The model under review builds one solid part; all positions refer to its coordinate system, in mm. Round coordinates to 2 decimals unless told otherwise and drop trailing zeros. Write each loop counter-clockwise with the first axis right and the second up, starting at its lowest first coordinate (ties: lowest second). Pieces come first, ordered by that corner, then holes. Notation, with made-up numbers: (48.5, -28) - (89.5, -28) arc R34 cw to (89.5, 4) - close; hole circle Ø2 at (19, 31.5). An arc over 180 degrees is marked (long way). Return JSON: item names as keys, results as strings.
from build123d import *

# Parameters (mm, degrees)
F0_R     = 17.5
F0_R_2   = 4.1
F0_R_3   = 3.375
F1_DEPTH = 10.75
F2_SIZE  = 3


with BuildPart() as f1:
    # F0 (on Top) → F1 (new body)
    with BuildSketch(Plane.XY):
        Circle(F0_R)
        with Locations((0, -8.725)):
            Circle(F0_R_2, mode=Mode.SUBTRACT)
        with Locations((-8.725, 0)):
            Circle(F0_R_3, mode=Mode.SUBTRACT)
        with Locations((8.725, 0)):
            Circle(F0_R_3, mode=Mode.SUBTRACT)
        with Locations((0, 8.725)):
            Circle(F0_R_2, mode=Mode.SUBTRACT)
    extrude(amount=F1_DEPTH)

    # F2
    f2_edges = [f1.edges().sort_by_distance(p)[0] for p in [
        (-4.1, 8.725, 10.75),
        (-4.1, -8.725, 10.75),
    ]]
    chamfer(f2_edges, length=F2_SIZE)


solid = f1.part
(1) Mouldability with a two-part tool opening along Y and no side actions: class faces 1 (the cylindrical face through (-0.889, 4.722, 3.821)), 2 (the flat face through (0, 0, 0)), 3 (the cylindrical face through (-5.5, 1, 5.3)), 4 (the cylindrical face through (-13.887, -10.648, 5.3)) as released by +Y, released by -Y, zero draft, split by the parting line, or undercut.
Filled in:
{"face 1": "undercut", "face 2": "zero draft", "face 3": "undercut", "face 4": "split by the parting line"}
(2) Add section C-C (x = 11). Write out the cut boundary in (y, z).
Filled in:
{"outline": "(-13.61, 0) - (-2.49, 0) - (-2.49, 10.75) - (-13.61, 10.75) - close; (2.49, 0) - (13.61, 0) - (13.61, 10.75) - (2.49, 10.75) - close"}
(3) Wall thickness on line 1 (Y direction, x = 0, z = 2.25) (3 decimals); line 2 (X direction, y = -0.5, z = 7.5); line 3 (X direction, y = -1.5, z = 3.25): over which ranges is each line inside the solid? List them lowest first.
Filled in:
{"line 1": "y = -17.5 to -12.825, -4.625 to 4.625, 12.825 to 17.5", "line 2": "x = -17.49 to -12.06, -5.39 to 5.39, 12.06 to 17.49", "line 3": "x = -17.44 to -11.75, -5.7 to 5.7, 11.75 to 17.44"}
(4) Add section D-D (z = 3.5). Write out the cut boundary in (x, y) (3 decimals), plus the area to 3 significant figures.
Filled in:
{"outline": "circle Ø35 at (0, 0); hole circle Ø6.75 at (-8.725, 0); hole circle Ø8.2 at (0, -8.725); hole circle Ø8.2 at (0, 8.725); hole circle Ø6.75 at (8.725, 0)", "area": "785 mm2"}
(5) Add section A-A (x = 0). Write out the cut boundary in (y, z) (3 decimals), plus the area to 3 significant figures.
Filled in:
{"outline": "(-17.5, 0) - (-12.825, 0) - (-12.825, 7.75) - (-15.825, 10.75) - (-17.5, 10.75) - close; (-4.625, 0) - (4.625, 0) - (4.625, 7.75) - (1.625, 10.75) - (-1.625, 10.75) - (-4.625, 7.75) - close; (12.825, 0) - (17.5, 0) - (17.5, 10.75) - (15.825, 10.75) - (12.825, 7.75) - close", "area": "182 mm2"}
(6) Add section B-B (y = 0). Write out the cut boundary in (x, z), plus the area to 3 significant figures.
Filled in:
{"outline": "(-17.5, 0) - (-12.1, 0) - (-12.1, 10.75) - (-17.5, 10.75) - close; (-5.35, 0) - (5.35, 0) - (5.35, 10.75) - (-5.35, 10.75) - close; (12.1, 0) - (17.5, 0) - (17.5, 10.75) - (12.1, 10.75) - close", "area": "231 mm2"}
